Verification items for the finished model (mm, model axes). A direction names the side the tool comes from. Round coordinates to 2 decimals unless told otherwise and drop trailing zeros. Order: outer loops, then holes, each group sorted by start corner. A loop starts at its lowest first (then second) coordinate and runs counter-clockwise, first axis right, second up. Notation, with made-up numbers: (-19, -4) -> (-12, -4) arc R29 ccw to (-12, 34) -> close; hole circle Ø3 at (25, 16). An arc over 180 degrees is marked (long way). Put each result on its own line as item: value.
```python
from build123d import *

# Parameters (mm, degrees)
F4_DEPTH = 3


with BuildPart() as f1:
    # F0 (on Top) → F1 (revolve)
    with BuildSketch(Plane.XY):
        Polygon((-41.3627406567, 2), (-40.1627406567, 2), (-7.2, 59.9687313223), (-8.4, 59.9687313223), (-10.2, 56.8032264431), align=None)
        Polygon((-10.2, 56.8032264431), (-8.4, 59.9687313223), (-10.2, 59.9687313223), align=None)
        Polygon((-8.4, 59.9687313223), (-7.2, 59.9687313223), (-7.2, 68.9687313223), (-10.2, 68.9687313223), (-10.2, 59.9687313223), align=None)
        Polygon((-42.5, 0), (-41.3, 0), (-40.1627406567, 2), (-41.3627406567, 2), align=None)
        Polygon((-45, 0), (-42.5, 0), (-41.3627406567, 2), (-45, 2), align=None)
    revolve(axis=Axis((0, 36.8, 0), (0, 1, 0)))

    # F3 (on offset) → F4 (join)
    with BuildSketch(Plane(origin=(0, 68.9687313223, 0), x_dir=(-1, 0, 0), z_dir=(0, 1, 0))):
        with BuildLine():
            ThreePointArc((6.2, -3.6606010435), (6.9455021417, -1.8973665961), (7.2, 0))
            ThreePointArc((7.2, 0), (6.9455021417, 1.8973665961), (6.2, 3.6606010435))
            Line((6.2, 3.6606010435), (6.2, 0))
            Line((6.2, 0), (6.2, -3.6606010435))
        make_face()
        with BuildLine():
            Line((-6.2, -3.6606010435), (-6.2, 3.6606010435))
            ThreePointArc((-6.2, 3.6606010435), (-7.2, 0), (-6.2, -3.6606010435))
        make_face()
    extrude(amount=-F4_DEPTH)


solid = f1.part
```
Item 1: Depth check by flat-ended pin: pin 1 Ø3.5 at (y, z) = (67.5, -1.5) entering from +X; pin 2 Ø1.1 at (x, z) = (-6.5, 1) entering from -Y; pin 3 Ø12 at (y, z) = (45, -10.5) entering from -X. Enter the tip coordinate at first touch or a pass-through.
Geometry check:
pin 1: x = 10.2
pin 2: y = 65.97
pin 3: x = -18.4
Item 2: Sectioned sample at B-B, the plane y = 10.5. Record the boundary of the cut face in (x, z), then the cut area to 3 significant figures.
Geometry check:
outline: circle Ø73.06 at (0, 0); hole circle Ø70.66 at (0, 0)
area: 271 mm2
Item 3: Material ranges on line 1 along Z through (x, y) = (0, 66.75); line 2 along Y through (x, z) = (-25.5, -34.5); line 3 along Z through (x, y) = (-30.5, 10.5), recorded low to high.
Geometry check:
line 1: -10.2 to -7.2, 7.2 to 10.2
line 2: 0 to 2
line 3: -20.1 to -17.83, 17.83 to 20.1
Item 4: Release check for a two-part mould opening along X. For faces 5 (the face through (6.2, 67, 0)), 6 (the face through (-20.765, 0.986, -39.923)), 7 (the face through (-7, 68.969, 0)) record: pulls with the +X half, pulls with the -X half, needs draft (parallel to the pull), parting line crosses it, or undercut.
Geometry check:
face 5: undercut
face 6: parting line crosses it
face 7: needs draft
Item 5: Sectioned sample at A-A, the plane y = 62.5. Record the boundary of the cut face in (x, z), then the cut area to 3 significant figures.
Geometry check:
outline: circle Ø20.4 at (0, 0); hole circle Ø14.4 at (0, 0)
area: 164 mm2
Item 6: Tool access check on faces 1 (the face through (-6.2, 67, 0)), 2 (the face through (19.8, 2, -36.5)), 3 (the face through (-19.8, 0, -36.5)), 4 (the face through (7.193, 64.532, 0.317)). Record the directions out of +Z, -Z, +X, -X, +Y, -Y that give a thin tool (end or side, any length) a straight path to the whole face; none if there is none.
Geometry check:
face 1: +Y, -Y
face 2: +Y
face 3: +Z, -Z, +X, -X, -Y
face 4: -Y
